Autodesk Inventor part; units mm, degrees
ref_plane "Work Plane1" through (3.81, 0, 8.636) normal (0, 0, 1) x (1, 0, 0)
ref_plane "Work Plane2" through (11.43, 0, 3.81) normal (0, 0, 1) x (1, 0, 0)
ref_plane "YZ Plane" through (0, 0, 0) normal (1, 0, 0) x (0, 1, 0)
sketch "Sketch1" plane through (0, 0, 0) normal (0, 0, 1) x (1, 0, 0)
  line L0 (0, 25.4) -> (60.96, 25.4)
  line L1 (60.96, 25.4) -> (60.96, 0)
  line L2 (60.96, 0) -> (0, 0)
  line L3 (0, 0) -> (0, 25.4)
  dimension "tmanifold_width" = 60.96
  dimension "tmanifold_depth" = 25.4
extrude "Extrusion1" add sketch "Sketch1" along normal blind 19.05
sketch "Sketch2" plane through (0, 0, 19.05) normal (0, 0, 1) x (1, 0, 0)
  line L0 (60.96, 25.4) -> (60.96, 0)
  line L1 (0, 25.4) -> (60.96, 25.4)
  line L2 (0, 0) -> (0, 25.4)
  line L3 (0, 12.7) -> (60.96, 12.7) construction
  line L4 (3.81, 17.78) -> (3.81, 12.7) construction
  line L5 (11.43, 7.62) -> (11.43, 12.7) construction
  point P0 (19.05, 17.78)
  point P1 (26.67, 7.62)
  point P2 (34.29, 17.78)
  point P3 (41.91, 7.62)
  point P4 (49.53, 17.78)
  point P5 (57.15, 7.62)
  dimension "d5" = 7.62
  dimension "d6" = 7.62
  dimension "d9" = 15.24
  dimension "d14" = 3.81
hole "top 10-32 ports" at (3.81, 17.78, 19.05) at (11.43, 7.62, 19.05) at (26.67, 7.62, 19.05) at (19.05, 17.78, 19.05) at (41.91, 7.62, 19.05) at (34.29, 17.78, 19.05) at (57.15, 7.62, 19.05) at (49.53, 17.78, 19.05) direction (0, 0, -1) diameter 3.9624 depth 6.604 countersink diameter 5.1054 countersink angle 90
sketch "Sketch3" plane through (0, 0, 0) normal (0, -1, 0) x (1, 0, 0)
  line L0 (60.96, 19.05) -> (0, 19.05)
  line L1 (60.96, 0) -> (0, 0)
  line L2 (1.8288, 12.446) -> (1.8288, 18.4785)
  line L3 (5.7912, 12.446) -> (5.7912, 18.4785)
  line L4 (5.7912, 12.446) -> (1.8288, 12.446)
  line L5 (9.4488, 12.446) -> (9.4488, 18.4785)
  line L6 (13.4112, 12.446) -> (13.4112, 18.4785)
  line L7 (13.4112, 12.446) -> (9.4488, 12.446)
  line L8 (3.81, 12.446) -> (3.81, 0) construction
  line L9 (11.43, 12.446) -> (11.43, 0) construction
  circle A0 centre (3.81, 8.636) radius 3.81 construction
  circle A1 centre (11.43, 3.81) radius 3.81 construction
  point P0 (19.05, 8.636)
  point P1 (26.67, 3.81)
  point P2 (34.29, 8.636)
  point P3 (41.91, 3.81)
  point P4 (49.53, 8.636)
  point P5 (57.15, 3.81)
  dimension "d22" = 7.62
  dimension "d25" = 15.24
  dimension "d78" = 8.636
  dimension "d79" = 3.81
hole "front 10-32 ports" at (3.81, 0, 8.636) at (11.43, 0, 3.81) at (19.05, 0, 8.636) at (26.67, 0, 3.81) at (34.29, 0, 8.636) at (41.91, 0, 3.81) at (49.53, 0, 8.636) at (57.15, 0, 3.81) direction (0, 1, 0) diameter 3.9624 depth 6.604 countersink diameter 5.1054 countersink angle 90
sketch "Sketch4" plane through (0, 25.4, 0) normal (0, 1, 0) x (1, 0, 0)
  circle A0 centre (3.81, -8.636) radius 2.5527
  circle A1 centre (11.43, -3.81) radius 2.5527
  circle A2 centre (19.05, -8.636) radius 2.5527
  circle A3 centre (26.67, -3.81) radius 2.5527
  circle A4 centre (34.29, -8.636) radius 2.5527
  circle A5 centre (41.91, -3.81) radius 2.5527
  circle A6 centre (49.53, -8.636) radius 2.5527
  circle A7 centre (57.15, -3.81) radius 2.5527
  dimension "d76" = 4.826
  dimension "d77" = 9.0197
hole "rear 10-32 ports" at (57.15, 25.4, 3.81) at (49.53, 25.4, 8.636) at (41.91, 25.4, 3.81) at (34.29, 25.4, 8.636) at (26.67, 25.4, 3.81) at (19.05, 25.4, 8.636) at (11.43, 25.4, 3.81) at (3.81, 25.4, 8.636) direction (0, -1, 0) diameter 3.9624 depth 6.604 countersink diameter 5.1054 countersink angle 90
sketch "Sketch5" plane through (0, 0, 0) normal (0, -1, 0) x (1, 0, 0)
  circle A0 centre (57.15, 3.81) radius 2.5527
  circle A1 centre (49.53, 8.636) radius 2.5527
  circle A2 centre (41.91, 3.81) radius 2.5527
  circle A3 centre (34.29, 8.636) radius 2.5527
  circle A4 centre (26.67, 3.81) radius 2.5527
  circle A5 centre (19.05, 8.636) radius 2.5527
  circle A6 centre (11.43, 3.81) radius 2.5527
  circle A7 centre (3.81, 8.636) radius 2.5527
hole "air channel thru" at (3.81, 0, 8.636) at (11.43, 0, 3.81) at (19.05, 0, 8.636) at (26.67, 0, 3.81) at (34.29, 0, 8.636) at (41.91, 0, 3.81) at (49.53, 0, 8.636) at (57.15, 0, 3.81) direction (0, 1, 0) diameter 1.016 end through all
sketch "Sketch6" plane through (0, 0, 19.05) normal (0, 0, 1) x (1, 0, 0)
  circle A0 centre (49.53, 17.78) radius 2.5527
  circle A1 centre (57.15, 7.62) radius 2.5527
  circle A2 centre (34.29, 17.78) radius 2.5527
  circle A3 centre (41.91, 7.62) radius 2.5527
  circle A4 centre (19.05, 17.78) radius 2.5527
  circle A5 centre (26.67, 7.62) radius 2.5527
  circle A6 centre (11.43, 7.62) radius 2.5527
  circle A7 centre (3.81, 17.78) radius 2.5527
ref_plane "Work Plane1" through (3.81, 0, 8.636) normal (0, 0, 1) x (1, 0, 0)
ref_plane "Work Plane2" through (11.43, 0, 3.81) normal (0, 0, 1) x (1, 0, 0)
hole "Hole5" at (3.81, 17.78, 19.05) at (19.05, 17.78, 19.05) at (34.29, 17.78, 19.05) at (49.53, 17.78, 19.05) direction (0, 0, -1) diameter 1.016 depth 10.414
hole "Hole6" at (11.43, 7.62, 19.05) at (26.67, 7.62, 19.05) at (41.91, 7.62, 19.05) at (57.15, 7.62, 19.05) direction (0, 0, -1) diameter 1.016 depth 15.24
sketch "Sketch7" plane through (0, 0, 0) normal (0, 0, -1) x (-1, 0, 0)
  line L0 (-1.8288, 6.604) -> (-1.8288, 0.5715)
  line L1 (-5.7912, 6.604) -> (-5.7912, 0.5715)
  line L2 (-3.302, 18.796) -> (-3.302, 6.604)
  line L3 (-4.318, 18.796) -> (-4.318, 6.604)
  line L4 (-1.8288, 18.796) -> (-1.8288, 24.8285)
  line L5 (-5.7912, 18.796) -> (-5.7912, 24.8285)
  line L6 (-1.8288, 18.796) -> (-5.7912, 18.796)
  line L7 (-5.7912, 6.604) -> (-1.8288, 6.604)
  line L8 (-8.8773, 0) -> (-13.9827, 0)
  line L9 (-13.4112, 0.5715) -> (-9.4488, 0.5715)
  line L10 (-13.4112, 6.604) -> (-13.4112, 0.5715)
  line L11 (-9.4488, 6.604) -> (-9.4488, 0.5715)
  line L12 (-10.922, 18.796) -> (-10.922, 6.604)
  line L13 (-11.938, 18.796) -> (-11.938, 6.604)
  line L14 (-9.4488, 18.796) -> (-13.4112, 18.796)
  line L15 (-18.542, 18.796) -> (-18.542, 6.604)
  line L16 (-19.558, 18.796) -> (-19.558, 6.604)
  line L17 (-21.0312, 6.604) -> (-17.0688, 6.604)
  line L18 (-28.6512, 6.604) -> (-24.6888, 6.604)
  line L19 (-36.2712, 6.604) -> (-32.3088, 6.604)
  line L20 (-31.7373, 0) -> (-36.8427, 0)
  line L21 (-43.8912, 6.604) -> (-39.9288, 6.604)
  line L22 (-51.5112, 6.604) -> (-47.5488, 6.604)
  line L23 (-49.022, 18.796) -> (-49.022, 6.604)
  line L24 (-50.038, 18.796) -> (-50.038, 6.604)
  line L25 (-49.022, 18.796) -> (-49.022, 6.604)
  line L26 (-50.038, 18.796) -> (-50.038, 6.604)
  line L27 (-33.782, 18.796) -> (-33.782, 6.604)
  line L28 (-33.782, 18.796) -> (-33.782, 6.604)
  line L29 (-32.3088, 6.604) -> (-32.3088, 0.5715)
  line L30 (-33.782, 18.796) -> (-33.782, 6.604)
  line L31 (-33.782, 18.796) -> (-33.782, 6.604)
  line L32 (-41.402, 18.796) -> (-41.402, 6.604)
  line L33 (-42.418, 18.796) -> (-42.418, 6.604)
  line L34 (-27.178, 18.796) -> (-27.178, 6.604)
  line L35 (-21.0312, 18.796) -> (-21.0312, 24.8285)
  line L36 (-27.178, 18.796) -> (-27.178, 6.604)
  line L37 (-42.418, 18.796) -> (-42.418, 6.604)
  line L38 (-36.2712, 18.796) -> (-36.2712, 24.8285)
  line L39 (-34.798, 18.796) -> (-34.798, 6.604)
  line L40 (-39.9288, 18.796) -> (-43.8912, 18.796)
  line L41 (-47.5488, 18.796) -> (-51.5112, 18.796)
  line L42 (-55.1688, 18.796) -> (-59.1312, 18.796)
  line L43 (-56.642, 18.796) -> (-56.642, 6.604)
  line L44 (-57.658, 18.796) -> (-57.658, 6.604)
  line L45 (-59.1312, 6.604) -> (-55.1688, 6.604)
  line L46 (-32.3088, 18.796) -> (-36.2712, 18.796)
  line L47 (-26.162, 18.796) -> (-26.162, 6.604)
  line L48 (-24.6888, 18.796) -> (-28.6512, 18.796)
  circle A0 centre (-49.53, 17.78) radius 2.5527
  circle A1 centre (-57.15, 7.62) radius 2.5527
  circle A2 centre (-34.29, 17.78) radius 2.5527
  circle A3 centre (-41.91, 7.62) radius 2.5527
  circle A4 centre (-19.05, 17.78) radius 2.5527
  circle A5 centre (-26.67, 7.62) radius 2.5527
  circle A6 centre (-11.43, 7.62) radius 2.5527
  circle A7 centre (-3.81, 17.78) radius 2.5527
  line L49 (-60.96, 25.4) -> (-60.96, 0)
  line L50 (0, 25.4) -> (-60.96, 25.4)
  line L51 (0, 0) -> (0, 25.4)
  line L52 (-60.96, 0) -> (0, 0)
  line L53 (-28.6512, 6.604) -> (-28.6512, 0.5715)
  line L54 (-24.6888, 6.604) -> (-24.6888, 0.5715)
  line L55 (-36.2712, 6.604) -> (-36.2712, 0.5715)
  line L56 (-39.9288, 6.604) -> (-39.9288, 0.5715)
  line L57 (-43.8912, 6.604) -> (-43.8912, 0.5715)
  line L58 (-47.5488, 6.604) -> (-47.5488, 0.5715)
  line L59 (-51.5112, 6.604) -> (-51.5112, 0.5715)
  line L60 (-55.1688, 6.604) -> (-55.1688, 0.5715)
  line L61 (-59.1312, 6.604) -> (-59.1312, 0.5715)
  line L62 (-39.9288, 18.796) -> (-39.9288, 24.8285)
  line L63 (-43.8912, 18.796) -> (-43.8912, 24.8285)
  line L64 (-51.5112, 18.796) -> (-51.5112, 24.8285)
  line L65 (-55.1688, 18.796) -> (-55.1688, 24.8285)
  line L66 (-59.1312, 18.796) -> (-59.1312, 24.8285)
  line L67 (-17.0688, 18.796) -> (-21.0312, 18.796)
  line L68 (-17.0688, 18.796) -> (-17.0688, 24.8285)
  line L69 (-17.0688, 6.604) -> (-17.0688, 0.5715)
  line L70 (-21.0312, 6.604) -> (-21.0312, 0.5715)
  line L71 (-13.4112, 18.796) -> (-13.4112, 24.8285)
  line L72 (-9.4488, 18.796) -> (-9.4488, 24.8285)
  circle A8 centre (-34.29, 17.78) radius 2.5527
  circle A9 centre (-19.05, 17.78) radius 2.5527
  circle A10 centre (-3.81, 17.78) radius 2.5527
  circle A11 centre (-11.43, 7.62) radius 2.5527
  circle A12 centre (-26.67, 7.62) radius 2.5527
  circle A13 centre (-41.91, 7.62) radius 2.5527
  circle A14 centre (-49.53, 17.78) radius 2.5527
  circle A15 centre (-57.15, 7.62) radius 2.5527
  line L73 (-32.3088, 18.796) -> (-32.3088, 24.8285)
  line L74 (-28.6512, 18.796) -> (-28.6512, 24.8285)
  line L75 (-24.6888, 18.796) -> (-24.6888, 24.8285)
  line L76 (-13.4112, 6.604) -> (-9.4488, 6.604)
  line L77 (-47.5488, 18.796) -> (-47.5488, 24.8285)
  line L78 (-60.96, 12.7) -> (0, 12.7) construction
  line L79 (-30.48, 25.4) -> (-30.48, 0) construction
  point P0 (-30.48, 12.7)
  point P1 (-15.24, 12.7)
  point P2 (-45.72, 12.7)
  dimension "d68" = 15.24
sketch "Sketch8" plane through (0, 0, 19.05) normal (0, 0, 1) x (1, 0, 0)
  circle A0 centre (49.53, 17.78) radius 2.5527
  circle A1 centre (57.15, 7.62) radius 2.5527
  circle A2 centre (34.29, 17.78) radius 2.5527
  circle A3 centre (41.91, 7.62) radius 2.5527
  circle A4 centre (19.05, 17.78) radius 2.5527
  circle A5 centre (26.67, 7.62) radius 2.5527
  circle A6 centre (11.43, 7.62) radius 2.5527
  circle A7 centre (3.81, 17.78) radius 2.5527
  line L0 (60.96, 25.4) -> (60.96, 0)
  line L1 (0, 25.4) -> (60.96, 25.4)
  line L2 (0, 0) -> (0, 25.4)
  line L3 (60.96, 0) -> (0, 0)
  line L4 (0, 12.7) -> (60.96, 12.7) construction
  line L5 (0, 12.7) -> (60.96, 12.7)
  line L6 (30.48, 0) -> (30.48, 25.4) construction
  line L7 (11.938, 18.796) -> (11.938, 6.604)
  line L8 (10.922, 18.796) -> (10.922, 6.604)
  line L9 (18.542, 18.796) -> (18.542, 6.604)
  line L10 (19.558, 18.796) -> (19.558, 6.604)
  line L11 (26.162, 18.796) -> (26.162, 6.604)
  line L12 (27.178, 18.796) -> (27.178, 6.604)
  line L13 (33.782, 18.796) -> (33.782, 6.604)
  line L14 (34.798, 18.796) -> (34.798, 6.604)
  line L15 (42.418, 18.796) -> (42.418, 6.604)
  line L16 (41.402, 18.796) -> (41.402, 6.604)
  line L17 (49.022, 18.796) -> (49.022, 6.604)
  line L18 (50.038, 18.796) -> (50.038, 6.604)
  point P0 (30.48, 12.7)
  point P1 (45.72, 12.7)
  point P2 (15.24, 12.7)
  dimension "d66" = 30.48
  dimension "d67" = 15.24
hole "Hole7" at (30.48, 12.7, 0) at (15.24, 12.7, 0) at (45.72, 12.7, 0) direction (0, 0, 1) diameter 3.302 depth 12.7 tip angle 118
properties part number "t-manifold"
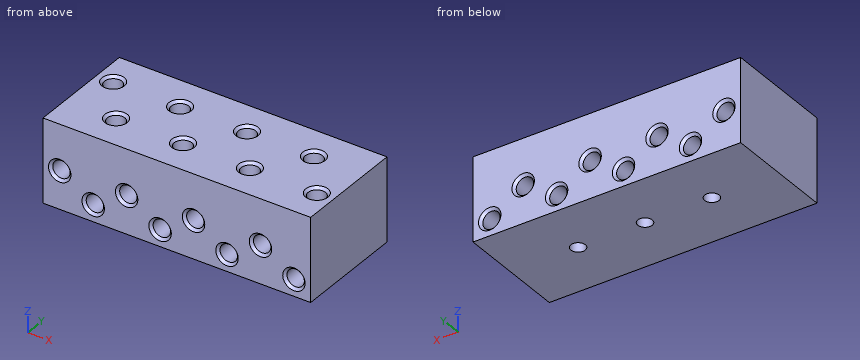
Design review of the part built by this model. Coordinates are the model's own, in mm. Give positions to 0.01 mm unless a question says otherwise; leave off trailing zeros. One line per question, with ' | ' between items. Start each with the question number.
1. Add section A-A (z = 2.75). Give the number of separate pieces and of enclosed holes in the cut face, plus the area to 3 significant figures.
2. To check wall thickness, follow L1, parallel to X at y = 3.25, z = 3.81; L2, parallel to X at y = 17.78, z = 15; L3, parallel to Z at x = 42, y = 16.75. State the ranges of each line that lie inside material, in increasing order.
3. Insertion check: P1, Ø1.2, axis at x = 41.91, y = 7.62, coming from the +Z side; P2, Ø1.2, axis at x = 26.5, z = 3.5, coming from the -Y side; P3, Ø2.5, axis at x = 41.91, y = 7.62, coming from the -Z side; P4, Ø2.5, axis at x = 41.91, z = 3.81, coming from the +Y side. Each pin has a flat end and moves straight along its axis. Give the tip position at first contact, or say it passes through.
Worked out:
1) separate pieces: 1 | enclosed holes: 3 | area: 1,340 mm²
2) L1: x = 0 to 9.45, 13.41 to 24.69, 28.65 to 39.93, 43.89 to 55.17, 59.13 to 60.96 | L2: x = 0 to 1.83, 5.79 to 17.07, 21.03 to 32.31, 36.27 to 47.55, 51.51 to 60.96 | L3: z = 0 to 3.31, 4.31 to 19.05
3) P1: stops at z = 12.45 | P2: stops at y = 6.6 | P3: stops at z = 0 | P4: stops at y = 18.8
